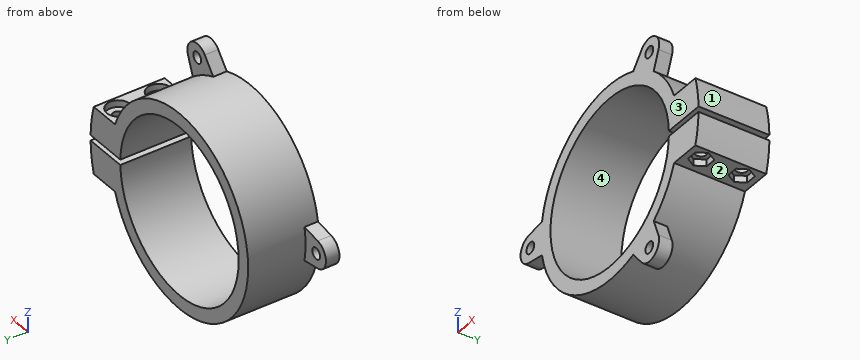
```python
from build123d import *

# Parameters (mm, degrees)
SKETCH_1_W               = 4
SKETCH_1_H               = 21
EXTRUDE_2_DEPTH          = 21
SKETCH_2_W               = 12.68061601
SKETCH_2_H               = 1.6
CUT_EXTRUDE_1_DEPTH      = 1
CUT_EXTRUDE_1_DEPTH_BACK = 22
SKETCH_4_R               = 1.65
CUT_EXTRUDE_2_DEPTH      = 40.05
CUT_EXTRUDE_3_DEPTH      = 2
SKETCH_6_R               = 3.45
SKETCH_6_R_2             = 1.65
CUT_EXTRUDE_4_DEPTH      = 2
SKETCH_7_R               = 1.65
EXTRUDE_3_DEPTH          = 4


with BuildPart() as part:
    # 草图1 → 旋转1 (revolve)
    with BuildSketch(Plane.XY):
        with Locations((27.05, 0)):
            Rectangle(SKETCH_1_W, SKETCH_1_H)
    revolve(axis=Axis((0, 0, 0), (0, 1, 0)))

    # 草图3 → 凸台-拉伸2 (add, through all)
    with BuildSketch(Plane(origin=(0, 10.5, 0), x_dir=(1, 0, 0), z_dir=(0, 1, 0))):
        with BuildLine():
            Line((27.274576074, 10), (36.274576074, 10))
            ThreePointArc((36.274576074, 10), (37.627714112, 0), (36.274576074, -10))
            Line((36.274576074, -10), (27.274576074, -10))
            Line((27.274576074, -10), (27.274576074, 10))
        make_face()
    extrude(amount=-EXTRUDE_2_DEPTH)

    # 草图2 → 切除-拉伸1 (cut, two sides)
    with BuildSketch(Plane(origin=(0, 10.5, 0), x_dir=(1, 0, 0), z_dir=(0, 1, 0))) as cut_extrude_1_sk:
        with Locations((31.287406107, 0)):
            Rectangle(SKETCH_2_W, SKETCH_2_H)
    extrude(amount=CUT_EXTRUDE_1_DEPTH, mode=Mode.SUBTRACT)
    extrude(cut_extrude_1_sk.sketch, amount=-CUT_EXTRUDE_1_DEPTH_BACK, mode=Mode.SUBTRACT)

    # 草图4 → 切除-拉伸2 (cut, through all)
    with BuildSketch(Plane.XY.offset(10)):
        with Locations((32.274576074, 6)):
            Circle(SKETCH_4_R)
        with Locations((32.274576074, -6)):
            Circle(SKETCH_4_R)
    extrude(amount=-CUT_EXTRUDE_2_DEPTH, mode=Mode.SUBTRACT)

    # 草图5 → 切除-拉伸3 (cut)
    with BuildSketch(Plane(origin=(0, 0, -10), x_dir=(-1, 0, 0), z_dir=(0, 0, -1))):
        Polygon((-30.65799532, 8.8), (-33.891156827, 8.8), (-35.507737581, 6), (-33.891156827, 3.2), (-30.65799532, 3.2), (-29.041414566, 6), align=None)
        Polygon((-30.65799532, -3.2), (-33.891156827, -3.2), (-35.507737581, -6), (-33.891156827, -8.8), (-30.65799532, -8.8), (-29.041414566, -6), align=None)
    extrude(amount=-CUT_EXTRUDE_3_DEPTH, mode=Mode.SUBTRACT)

    # 草图6 → 切除-拉伸4 (cut)
    with BuildSketch(Plane.XY.offset(10)):
        with Locations((32.274576074, -6)):
            Circle(SKETCH_6_R)
        with Locations((32.274576074, -6)):
            Circle(SKETCH_6_R_2, mode=Mode.SUBTRACT)
        with Locations((32.274576074, 6)):
            Circle(SKETCH_6_R)
        with Locations((32.274576074, 6)):
            Circle(SKETCH_6_R_2, mode=Mode.SUBTRACT)
    extrude(amount=-CUT_EXTRUDE_4_DEPTH, mode=Mode.SUBTRACT)

    # 草图7 → 凸台-拉伸3 (add)
    with BuildSketch(Plane.XZ.offset(10.5)):
        with BuildLine():
            Line((-34.211268637, 4.096977397), (-28.616472529, 5))
            ThreePointArc((-28.616472529, 5), (-29.05, 0), (-28.616472529, -5))
            Line((-28.616472529, -5), (-34.211268637, -4.096977397))
            ThreePointArc((-34.211268637, -4.096977397), (-37.7, 0), (-34.211268637, 4.096977397))
        make_face()
        with Locations((-33.55, 0)):
            Circle(SKETCH_7_R, mode=Mode.SUBTRACT)
        with BuildLine():
            Line((20.653720823, 27.579339037), (18.638363283, 22.282592177))
            ThreePointArc((18.638363283, 22.282592177), (14.525, 25.15803798), (9.978109246, 27.282592177))
            Line((9.978109246, 27.282592177), (13.557547814, 31.676316433))
            ThreePointArc((13.557547814, 31.676316433), (18.85, 32.649157723), (20.653720823, 27.579339037))
        make_face()
        with Locations((16.775, 29.055152297)):
            Circle(SKETCH_7_R, mode=Mode.SUBTRACT)
        with BuildLine():
            Line((13.557547814, -31.676316433), (9.978109246, -27.282592177))
            ThreePointArc((9.978109246, -27.282592177), (14.525, -25.15803798), (18.638363283, -22.282592177))
            Line((18.638363283, -22.282592177), (20.653720823, -27.579339037))
            ThreePointArc((20.653720823, -27.579339037), (18.85, -32.649157723), (13.557547814, -31.676316433))
        make_face()
        with Locations((16.775, -29.055152297)):
            Circle(SKETCH_7_R, mode=Mode.SUBTRACT)
    extrude(amount=-EXTRUDE_3_DEPTH)


solid = part.part
```
Verification items for the finished model (mm, model axes). Face numbers are marked on the shaded views. Coordinates: 2 decimals unless noted, no trailing zeros. Write each loop counter-clockwise with the first axis right and the second up, starting at its lowest first coordinate (ties: lowest second). Pieces come first, ordered by that corner, then holes. Notation, with made-up numbers: (14.25, 29.25) - (51.25, 29.25) arc R28 cw to (51.25, 59.25) - close; hole circle Ø7 at (-13, 56). An arc over 180 degrees is marked (long way). Write item = value, one per line.
Q1. Cross-section at C-C (z = -21). Enter the section's corners in (x, y), plus the area to 3 significant figures.
Answer:
outline = (-20.07, -10.5) - (-13.66, -10.5) - (-13.66, 10.5) - (-20.07, 10.5) - close; (13.66, -10.5) - (20.07, -10.5) - (20.07, 10.5) - (13.66, 10.5) - close
area = 269 mm²
Q2. Mould release check, pull along Z, two halves, no side actions. Record for the marked faces 1, 2, 3 and 4: released by +Z, released by -Z, zero draft, split by the parting line, or undercut.
Answer:
face_1 = released by +Z
face_2 = released by -Z
face_3 = zero draft
face_4 = undercut
Q3. Cross-section at B-B (y = 0.25). Enter the section's corners in (x, z), plus the area to 3 significant figures.
Answer:
outline = (25.04, -0.8) arc R25.05 cw (long way) to (25.04, 0.8) - (37.62, 0.8) arc R37.63 ccw to (36.27, 10) - (27.27, 10) arc R29.05 ccw (long way) to (27.27, -10) - (36.27, -10) arc R37.63 ccw to (37.62, -0.8) - close
area = 834 mm²
Q4. Go/stop test with flat-tipped pins: pin 1 Ø4.5 at (x, y) = (32.27, -6) entering from +Z; pin 2 Ø3 at (x, z) = (13, 20.5) entering from -Y; pin 3 Ø2 at (x, z) = (-21.5, 6.5) entering from +Y; pin 4 Ø1.7 at (x, y) = (31.5, -5) entering from -Z. Record where each tip stops, or that it passes through.
Answer:
pin_1 = 8
pin_2 = -10.5
pin_3 = through
pin_4 = -8
Q5. Material ranges on L1, parallel to Z at x = 0, y = -0.25; L2, parallel to Z at x = 32, y = -9; L3, parallel to X at y = 9.25, z = -13.5, recorded low to high. Write a range as from..to.
Answer:
L1 = -29.05..-25.05, 25.05..29.05
L2 = -10..-0.8, 0.8..8
L3 = -25.72..-21.1, 21.1..25.72
Q6. Cross-section at A-A (x = 0). Enter the section's corners in (y, z), plus the area to 3 significant figures.
Answer:
outline = (-10.5, -29.05) - (10.5, -29.05) - (10.5, -25.05) - (-10.5, -25.05) - close; (-10.5, 25.05) - (10.5, 25.05) - (10.5, 29.05) - (-10.5, 29.05) - close
area = 168 mm²
